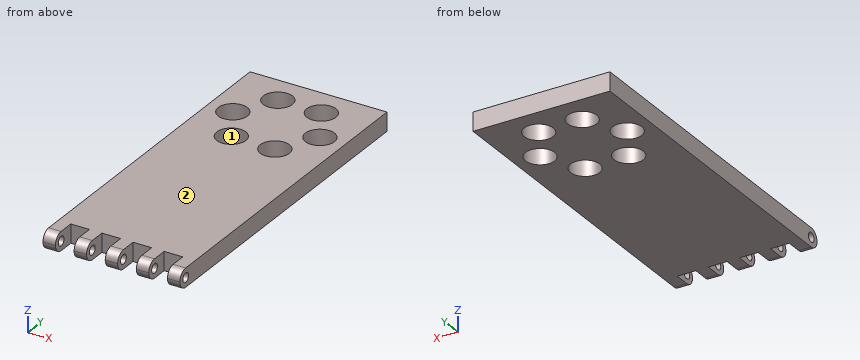
from build123d import *

# Parameters (mm, degrees)
SKETCH1_W              = 44
SKETCH1_H              = 100
BOSS_EXTRUDE1_DEPTH    = 6
SKETCH3_R              = 4.7
CUT_EXTRUDE4_DEPTH     = 10
SKETCH4_W              = 4
SKETCH4_H              = 6
BOSS_EXTRUDE2_DEPTH    = 8
FILLET1_R              = 3
LPATTERN1_COUNT        = 5
LPATTERN1_PITCH        = 10
FILLET1_OF_LPATTERN1_R = 3
SKETCH5_R              = 1.5
CUT_EXTRUDE5_DEPTH     = 74.047929471


with BuildPart() as part:
    # Sketch1 → Boss-Extrude1 (new body)
    with BuildSketch(Plane.XY):
        Rectangle(SKETCH1_W, SKETCH1_H)
    extrude(amount=BOSS_EXTRUDE1_DEPTH)

    # Sketch3 → Cut-Extrude4 (cut)
    with BuildSketch(Plane.XY.offset(6)):
        with Locations((-7.002612265, 40.123358619)):
            Circle(SKETCH3_R)
        with Locations((6.997387735, 40.123358619)):
            Circle(SKETCH3_R)
        with Locations((13.997387735, 27.999002966)):
            Circle(SKETCH3_R)
        with Locations((6.997387735, 15.874647313)):
            Circle(SKETCH3_R)
        with Locations((-7.002612265, 15.874647313)):
            Circle(SKETCH3_R)
        with Locations((-14.002612265, 27.999002966)):
            Circle(SKETCH3_R)
    extrude(amount=-CUT_EXTRUDE4_DEPTH, mode=Mode.SUBTRACT)

    # Sketch4 → Boss-Extrude2 (add)
    with BuildSketch(Plane.XZ.offset(50)):
        with Locations((-20, 3)):
            Rectangle(SKETCH4_W, SKETCH4_H)
    boss_extrude2 = extrude(amount=BOSS_EXTRUDE2_DEPTH)

    # Fillet1
    fillet1_edges = [part.edges().sort_by_distance(p)[0] for p in [
        (-20, -58, 6),
        (-20, -58, 0),
    ]]
    fillet(fillet1_edges, radius=FILLET1_R - 0.0001)  # a hair under: the kernel refuses the full size

    # LPattern1: Boss-Extrude2 ×5
    with Locations(*[(i * LPATTERN1_PITCH, 0, 0) for i in range(1, LPATTERN1_COUNT)]):
        add(boss_extrude2)

    # Fillet1 of LPattern1
    fillet1_of_lpattern1_edges = [part.edges().sort_by_distance(p)[0] for p in [
        (-10, -58, 6),
        (-10, -58, 0),
        (0, -58, 6),
        (0, -58, 0),
        (10, -58, 6),
        (10, -58, 0),
        (20, -58, 6),
        (20, -58, 0),
    ]]
    fillet(fillet1_of_lpattern1_edges, radius=FILLET1_OF_LPATTERN1_R - 0.0001)  # a hair under: the kernel refuses the full size

    # Sketch5 → Cut-Extrude5 (cut, through all)
    with BuildSketch(Plane.ZY.offset(22)):
        with Locations(Location((3, -55, 0), (0, 0, 270))):
            Circle(SKETCH5_R)
    extrude(amount=-CUT_EXTRUDE5_DEPTH, mode=Mode.SUBTRACT)


solid = part.part
Verification items for the finished model (mm, model axes). Face numbers are marked on the shaded views. Coordinates: 2 decimals unless noted, no trailing zeros. Loops run counter-clockwise (first coordinate to the right, second up) from the corner with the lowest first, then second, coordinate; pieces in that order, holes last. Notation, with made-up numbers: (82, -17) -> (141, -17) arc R24 ccw to (141, 20) -> close; hole circle Ø9 at (14, 87.25). An arc over 180 degrees is marked (long way). Write each question's results on one line, items separated by ' | '.
Item 1: Gauge pin test, flat ends, axial feed: pin 1 (3 mm diameter, centred on x = -16, z = 3, fed in from -Y); pin 2 (5.5 mm diameter, centred on x = -7, y = 15.87, fed in from -Z). Record the tip position at first contact, or that the pin passes through.
Found:
pin 1: stops at y = -50 | pin 2: passes through
Item 2: Mould release check, pull along X, two halves, no side actions. Record for the marked faces 1 and 2: +X half, -X half, draft (parallel to the pull), parting line (faces both ways), or undercut.
Found:
face 1: undercut | face 2: draft
Item 3: Section check C-C, the plane x = -5. Enter the section's corners in (y, z).
Found:
outline: (-50, 0) -> (11.62, 0) -> (11.62, 6) -> (-50, 6) -> close; (20.13, 0) -> (35.87, 0) -> (35.87, 6) -> (20.13, 6) -> close; (44.38, 0) -> (50, 0) -> (50, 6) -> (44.38, 6) -> close
Item 4: Material ranges on L1, parallel to Y at x = 7, z = 1.2; L2, parallel to Z at x = 1, y = -55; L3, parallel to X at y = -51, z = 4.7, recorded low to high.
Found:
L1: y = -50 to 11.17, 20.57 to 35.42, 44.82 to 50 | L2: z = 0 to 1.5, 4.5 to 6 | L3: x = -22 to -18, -12 to -8, -2 to 2, 8 to 12, 18 to 22
Item 5: Section check B-B, the plane x = 6.5. Enter the section's corners in (y, z).
Found:
outline: (-50, 0) -> (11.2, 0) -> (11.2, 6) -> (-50, 6) -> close; (20.55, 0) -> (35.45, 0) -> (35.45, 6) -> (20.55, 6) -> close; (44.8, 0) -> (50, 0) -> (50, 6) -> (44.8, 6) -> close
Item 6: Section check A-A, the plane x = -16. Enter the section's corners in (y, z), plus the area to 3 significant figures.
Found:
outline: (-50, 0) -> (23.74, 0) -> (23.74, 6) -> (-50, 6) -> close; (32.25, 0) -> (50, 0) -> (50, 6) -> (32.25, 6) -> close | area: 549 mm2
